Geometry check sheet. Reference: the model listing, model coordinates, mm. Give positions to 0.01 mm unless a question says otherwise; leave off trailing zeros. Order: outer loops, then holes, each group sorted by start corner. A loop starts at its lowest first (then second) coordinate and runs counter-clockwise, first axis right, second up.
from build123d import *

# Parameters (mm, degrees)
CROQUIS1_W              = 77
CROQUIS1_H              = 61
SALIENTE_EXTRUIR1_DEPTH = 5
CROQUIS2_R              = 2
CORTAR_EXTRUIR1_DEPTH   = 5
REDONDEO2_R             = 2
REDONDEO3_R             = 2
REDONDEO4_R             = 2


with BuildPart() as part:
    # Croquis1 → Saliente-Extruir1 (new body)
    with BuildSketch(Plane(origin=(0, 0, 0), x_dir=(0, 0, -1), z_dir=(1, 0, 0))):
        Rectangle(CROQUIS1_W, CROQUIS1_H)
    extrude(amount=SALIENTE_EXTRUIR1_DEPTH)

    # Croquis2 → Cortar-Extruir1 (cut)
    with BuildSketch(Plane(origin=(5, 0, 0), x_dir=(0, 0, -1), z_dir=(1, 0, 0))):
        with Locations((-34.75, 25.5)):
            Circle(CROQUIS2_R)
        with Locations((-34.75, -25.5)):
            Circle(CROQUIS2_R)
        with Locations((34.75, 25.5)):
            Circle(CROQUIS2_R)
        with Locations((34.75, -25.5)):
            Circle(CROQUIS2_R)
    extrude(amount=-CORTAR_EXTRUIR1_DEPTH, mode=Mode.SUBTRACT)

    # Redondeo2
    redondeo2_edges = [part.edges().sort_by_distance(p)[0] for p in [
        (2.5, 30.5, 38.5),
    ]]
    fillet(redondeo2_edges, radius=REDONDEO2_R)

    # Redondeo3
    redondeo3_edges = [part.edges().sort_by_distance(p)[0] for p in [
        (2.5, 30.5, -38.5),
    ]]
    fillet(redondeo3_edges, radius=REDONDEO3_R)

    # Redondeo4
    redondeo4_edges = [part.edges().sort_by_distance(p)[0] for p in [
        (2.5, -30.5, -38.5),
        (2.5, -30.5, 38.5),
    ]]
    fillet(redondeo4_edges, radius=REDONDEO4_R)


solid = part.part
Item 1: Gauge pin test, flat end, axial feed: pin 1 (2.5 mm diameter, centred on y = -25.5, z = 34.75, fed in from -X). Record the tip position at first contact, or that the pin passes through.
Reported:
pin 1: passes through
Item 2: Scan lines: L1, parallel to Y at x = 2.9, z = 34.75; L2, parallel to Z at x = 2.1, y = 25; L3, parallel to Z at x = 4.4, y = -24. Record each from-to range of solid material in increasing order.
Reported:
L1: y = -30.5 to -27.5, -23.5 to 23.5, 27.5 to 30.5
L2: z = -38.5 to -36.69, -32.81 to 32.81, 36.69 to 38.5
L3: z = -38.5 to -36.07, -33.43 to 33.43, 36.07 to 38.5
Item 3: Sectioned sample at A-A (z = 34.75). Enter the section's corners in (x, y).
Reported:
outline: (0, -30.5) - (5, -30.5) - (5, -27.5) - (0, -27.5) - close; (0, -23.5) - (5, -23.5) - (5, 23.5) - (0, 23.5) - close; (0, 27.5) - (5, 27.5) - (5, 30.5) - (0, 30.5) - close
Item 4: Sectioned sample at B-B (y = 25.5). Enter the section's corners in (x, z), and give its area (3 significant figures).
Reported:
outline: (0, -38.5) - (5, -38.5) - (5, -36.75) - (0, -36.75) - close; (0, -32.75) - (5, -32.75) - (5, 32.75) - (0, 32.75) - close; (0, 36.75) - (5, 36.75) - (5, 38.5) - (0, 38.5) - close
area: 345 mm2
Item 5: Draft check along Y on faces 1 (the cylindrical face through (2.535, 24.734, 32.903)), 2 (the flat face through (5, 0, 1)), 3 (the flat face through (2, 30.5, 1)). Enter one of: released by +Y, released by -Y, zero draft, split by the parting line, or undercut.
Reported:
face 1: undercut
face 2: zero draft
face 3: released by +Y
